Solid Edge part; units mm, degrees
sketch "Sketch1" plane through (0, 0, 0) normal (0, -1, 0) x (1, 0, 0)
  line L0 (21.2, 4.4667) -> (41.2, 4.4667)
  line L1 (41.2, 4.4667) -> (41.2, 44.4667)
  line L2 (41.2, 44.4667) -> (21.2, 44.4667)
  line L3 (21.2, 44.4667) -> (21.2, 4.4667)
  dimension "D1" = 21.2
  dimension "D2" = 41.2
extrude "Protrusion1" add sketch "Sketch1" against normal blind 15
sketch "Sketch2" plane through (31.2, 0, 24.4667) normal (0, -1, 0) x (1, 0, 0)
  circle A0 centre (0, 10) radius 7
extrude "ExtrudedCutout_1" cut sketch "Sketch2" against normal blind 10
sketch "Sketch3" plane through (21.2, 7.5, 24.4667) normal (-1, 0, 0) x (0, -1, 0)
  line L0 (7.5, 13.5) -> (2.5, 13.5)
  arc A0 (2.5, 13.5) -> (2.5, 6) centre (2.5, 9.75) ccw
  line L1 (2.5, 6) -> (7.5, 6)
  line L2 (7.5, 13.5) -> (7.5, 6)
  dimension "D1" = 7.5
extrude "Cutout1" cut sketch "Sketch3" against normal through all
sketch "Sketch4" plane through (31.2, 15, 24.4667) normal (0, 1, 0) x (-1, 0, 0)
  line L0 (-10, 20) -> (-4, 20)
  line L1 (-4, 20) -> (-4, -20)
  line L2 (-4, -20) -> (-10, -20)
  line L3 (-10, -20) -> (-10, 20)
  dimension "D1" = 10
extrude "Cutout2" cut sketch "Sketch4" against normal through all
sketch "Sketch5" plane through (28.2, 7.5, 4.4667) normal (0, 0, -1) x (1, 0, 0)
  line L0 (5.8777, 7.5) -> (5.8777, 2.5)
  arc A0 (5.8777, 2.5) -> (-1.6223, 2.5) centre (2.1277, 2.5) cw
  line L1 (-1.6223, 2.5) -> (-1.6223, 7.5)
  line L2 (5.8777, 7.5) -> (-1.6223, 7.5)
  dimension "D1" = 1.6223
  dimension "D2" = 5.8777
extrude "Cutout3" cut sketch "Sketch5" against normal up to next
sketch "Sketch6" plane through (28.2, 15, 24.4667) normal (0, 1, 0) x (-1, 0, 0)
  line L0 (-7, -20) -> (7, -20)
  line L1 (7, -20) -> (7, -1)
  line L2 (7, -1) -> (-7, -1)
  line L3 (-7, -1) -> (-7, -20)
  dimension "D1" = 7
extrude "Cutout4" cut sketch "Sketch6" against normal up to next
sketch "Sketch7" plane through (28.2, 15, 33.9667) normal (0, 1, 0) x (-1, 0, 0)
  line L0 (-39.04, 20.5) -> (-39.04, -19.5)
  line L1 (-39.04, -19.5) -> (50.96, -19.5)
  line L2 (50.96, 20.5) -> (50.96, -19.5)
  line L3 (-39.04, 20.5) -> (50.96, 20.5)
  dimension "D1" = 39.04
  dimension "D2" = 39.04
  dimension "D3" = 50.96
extrude "ExtrudedProtrusion_2" add sketch "Sketch7" along normal blind 3
sketch "Sketch8" plane through (19.24, 18, 34.4667) normal (0, 1, 0) x (-1, 0, 0)
  circle A0 centre (-43, 15) radius 1.65
  circle A1 centre (37, -15) radius 1.65
  dimension "D1" = 43
extrude "Cutout5" cut sketch "Sketch8" against normal through all
sketch "Sketch9" plane through (19.24, 18, 34.4667) normal (0, 1, 0) x (-1, 0, 0)
  circle A0 centre (-43, 15) radius 3.55
  circle A1 centre (37, -15) radius 3.55
extrude "ExtrudedCutout_9" cut sketch "Sketch9" against normal blind 0.5
Geometry: final body of the model. Coordinates: model frame, mm. A direction names the side the tool comes from. Coordinates: 2 decimals unless noted, no trailing zeros. Write each loop counter-clockwise with the first axis right and the second up, starting at its lowest first coordinate (ties: lowest second). Pieces come first, ordered by that corner, then holes. Notation, with made-up numbers: M -39,73.5 L -31,73.5 A23 cw -31,83.5 Z; hole C 29,45 d5. An arc over 180 degrees is marked long. Use CSV: the item, a comma, the result in double quotes. Start each with the question number.
1. Cut plane B-B on y = 3.25. Return the cut outline in (x, z).
2. Reachability of faces 4 (the face through (27.41, 6.04, 40.35)), 5 (the face through (30.25, 8.75, 25.66)), 6 (the face through (28, 9, 23.467)), 7 (the face through (23, 2, 37.967)), 8 (the face through (65.06, 17.75, 47.31)) from +Z, -Z, +X, -X, +Y, -Y: full face, straight path, thin tool, end or side. Return the list, or none.
3. Ray query, probe 1 along Y at (x, z) = (55.5, 51); probe 2 along X at (y, z) = (5, 27); probe 3 along Z at (x, y) = (31.2, 7.5). Return the intervals inside material, ascending.
4. Mould query, pull axis X, two halves, no side actions, for faces 1 (the face through (35.2, 11, 34)), 2 (the face through (-18.647, 16.267, 20.858)), 3 (the face through (28, 7, 44.467)). Classes: pulls with the +X half, pulls with the -X half, needs draft (parallel to the pull), parting line crosses it, or undercut.
5. Cut plane A-A on x = 62.24. Return the cut outline in (y, z), plus the area to 3 significant figures.
6. First-contact query: P1, Ø5.5, axis at x = -17.76, z = 19.47, coming from the -Y side; P2, Ø3.5, axis at x = 61.5, z = 48.5, coming from the +Y side; P3, Ø10, axis at y = 4, z = 27.5, coming from the -X side; P4, Ø2, axis at x = 62.24, z = 49.47, coming from the -Y side (3 decimals). Flat tips, straight axial feed; report the tip coordinate or a pass-through.
7. Cut plane C-C on z = 22. Return the cut outline in (x, y), plus the area to 3 significant figures.
8. Cut plane D-D on x = 31.2. Return the cut outline in (y, z), plus the area to 3 significant figures.
Entries:
1,outline,"M 21.2,23.47 L 26.58,23.47 L 26.58,29.21 A7 cw 25.46,30.47 L 21.2,30.47 Z; M 21.2,37.97 L 25.14,37.97 A7 cw 35.2,40.21 L 35.2,44.47 L 21.2,44.47 Z; M 34.08,23.47 L 35.2,23.47 L 35.2,28.72 A7 cw 34.08,28.09 Z"
2,face 4,"-Y"
2,face 5,"-Z, -Y"
2,face 6,"-Z, +X, -X, -Y"
2,face 7,"+X, -X, -Y"
2,face 8,"+Y"
3,probe 1,"15 to 18"
3,probe 2,"21.2 to 26.58, 34.08 to 35.2"
3,probe 3,"41.47 to 44.47"
4,face 1,"pulls with the +X half"
4,face 2,"undercut"
4,face 3,"needs draft"
5,outline,"M 15,14.47 L 18,14.47 L 18,45.92 L 17.5,45.92 L 17.5,47.82 L 15,47.82 Z; M 15,51.12 L 17.5,51.12 L 17.5,53.02 L 18,53.02 L 18,54.47 L 15,54.47 Z"
5,area,"108 mm²"
6,P1,"y = 15"
6,P2,"y = 17.5"
6,P3,"x = 21.2"
6,P4,"through"
7,outline,"M -22.76,15 L 67.24,15 L 67.24,18 L -15.27,18 L -15.27,17.5 L -20.25,17.5 L -20.25,18 L -22.76,18 Z"
7,area,"268 mm²"
8,outline,"M 0,41.47 L 10,41.47 L 10,27.47 L 8.65,27.47 L 8.65,23.47 L 15,23.47 L 15,14.47 L 18,14.47 L 18,54.47 L 15,54.47 L 15,44.47 L 0,44.47 Z"
8,area,"260 mm²"
